Geometry: final body of the model. Coordinates: model frame, mm. A direction names the side the tool comes from. Coordinates: 2 decimals unless noted, no trailing zeros. Loops run counter-clockwise (first coordinate to the right, second up) from the corner with the lowest first, then second, coordinate; pieces in that order, holes last. Notation, with made-up numbers: (-39.5, -32) -> (-26.5, -32) arc R22 cw to (-26.5, -5) -> close; hole circle Ø7 at (8, 24). An arc over 180 degrees is marked (long way). One line per item, written item: value. Start each with the question number.
Autodesk Inventor part; units mm, degrees
ref_plane "Work Plane1" through (0, 0, -7) normal (0, 0, 1) x (1, 0, 0)
ref_plane "YZ Plane" through (0, 0, 0) normal (1, 0, 0) x (0, 1, 0)
ref_plane "XZ Plane" through (0, 0, 0) normal (0, 1, 0) x (-1, 0, 0)
sketch "Sketch1" plane through (0, 0, 0) normal (0, 1, 0) x (-1, 0, 0)
  circle A0 centre (0, 0) radius 7
  dimension "d0" = 14
extrude "Extrusion1" add sketch "Sketch1" along normal blind 30
sketch "Sketch2" plane through (0, 0, 0) normal (0, -1, 0) x (1, 0, 0)
  point P0 (0, 0)
ref_plane "Work Plane1" through (0, 0, -7) normal (0, 0, 1) x (1, 0, 0)
sketch "Sketch3" plane through (0, 0, -7) normal (0, 0, 1) x (1, 0, 0)
  line L0 (0, 5) -> (0, 5)
  line L1 (-2.5, 7.5) -> (-2.5, 22.5)
  line L2 (0, 25) -> (0, 25)
  line L3 (2.5, 22.5) -> (2.5, 7.5)
  line L4 (7, 0) -> (-7, 0)
  arc A0 (0, 5) -> (2.5, 7.5) centre (0, 7.5) ccw
  arc A1 (-2.5, 7.5) -> (0, 5) centre (0, 7.5) ccw
  arc A2 (0, 25) -> (-2.5, 22.5) centre (0, 22.5) ccw
  arc A3 (2.5, 22.5) -> (0, 25) centre (0, 22.5) ccw
  point P0 (0, 0)
  point P1 (2.5, 5)
  point P2 (2.5, 25)
  point P3 (0, 5)
  point P4 (0, 25)
  dimension "d3" = 5
  dimension "d4" = 20
  dimension "d5" = 5
  dimension "d6" = 2.5
  dimension "d7" = 2.5
extrude "Extrusion2" add sketch "Sketch3" along normal blind 1 and the other way blind 2
sketch "Sketch4" plane through (0, 0, 0) normal (0, -1, 0) x (1, 0, 0)
  circle A0 centre (0, 0) radius 3
  dimension "d12" = 6
extrude "Extrusion3" cut sketch "Sketch4" against normal blind 8
chamfer "Chamfer1" distance 0.5 angle 45 1 edges at (7, 0, 0)
thread "Thread1"
properties part number "inputshaft nmrv50"
1. Pin query (flat end, axial travel): pin 1 Ø1.5 at (y, z) = (26, 2) entering from +X; pin 2 Ø1 at (x, y) = (4, 26) entering from -Z; pin 3 Ø2 at (y, z) = (14.5, -8) entering from +X. Return the tip coordinate at first contact, or that it passes through.
2. Line query: L1, parallel to Z at x = 0, y = 3.5; L2, parallel to Y at x = -2.25, z = 1.5; L3, parallel to Z at x = 0, y = 6.25. Output: solid intervals per line, ascending. Write a range as [from, to].
3. Set-up query: faces 1 (the face through (0, 25, -8)), 2 (the face through (-2.5, 15, -8)), 3 (the face through (-3, 4, 0)). Return all of +Z, -Z, +X, -X, +Y, -Y with unobstructed straight access to the full face (end or side cutting, diameter ignored); none if empty.
4. Section C-C on z = 0. Return the cut outline in (x, y).
5. Section A-A on x = 0. Return the cut outline in (y, z), plus the area to 3 significant figures.
6. Section D-D on y = 28. Return the cut outline in (x, z).
7. Draft query along X for faces 4 (the face through (0, 5, -8)), 5 (the face through (0, 8, 0)), 6 (the face through (0, 15, -9)). Return one class per face: released by +X, released by -X, zero draft, split by the parting line, or undercut.
8. Section B-B on y = 4. Return the cut outline in (x, z), plus the area to 3 significant figures.
Checks:
1. pin 1: x = 6.89
1. pin 2: z = -6.06
1. pin 3: x = 2.5
2. L1: [-7, -3], [3, 7]
2. L2: [8, 30]
2. L3: [-9, -3], [3, 7]
3. face 1: -Z, +Y
3. face 2: -Z, -X, +Y, -Y
3. face 3: -Y
4. outline: (-7, 0.5) -> (-6.5, 0) -> (-3, 0) -> (-3, 8) -> (3, 8) -> (3, 0) -> (6.5, 0) -> (7, 0.5) -> (7, 30) -> (-7, 30) -> close
5. outline: (0, -6.5) -> (0.5, -7) -> (5, -7) -> (5, -9) -> (25, -9) -> (25, -7) -> (30, -7) -> (30, 7) -> (0.5, 7) -> (0, 6.5) -> (0, 3) -> (8, 3) -> (8, -3) -> (0, -3) -> close
5. area: 412 mm²
6. outline: circle Ø14 at (0, 0)
7. face 4: split by the parting line
7. face 5: undercut
7. face 6: zero draft
8. outline: circle Ø14 at (0, 0); hole circle Ø6 at (0, 0)
8. area: 126 mm²
